Geometry: final body of the model. Coordinates: model frame, mm. Face numbers are marked on the shaded views. A direction names the side the tool comes from. Give positions to 0.01 mm unless a question says otherwise; leave off trailing zeros. Loops run counter-clockwise (first coordinate to the right, second up) from the corner with the lowest first, then second, coordinate; pieces in that order, holes last.
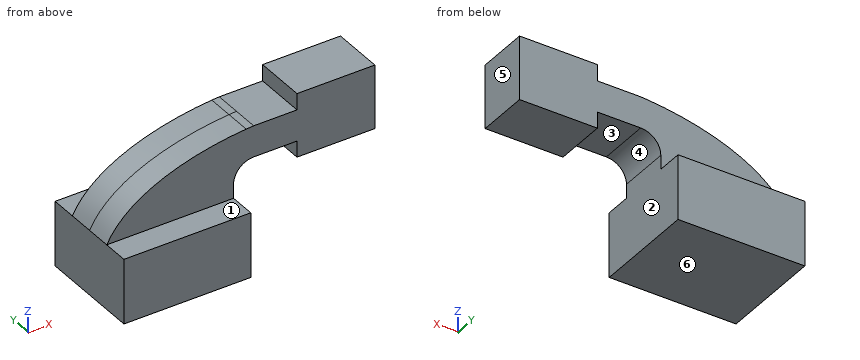
```python
from build123d import *

# Parameters (mm, degrees)
F1_DEPTH = 12.5
F2_DEPTH = 25
F0_W     = 18.6651162803
F0_H     = 7.8595249355
F0_H_2   = 15
F0_H_3   = 7.7596530318
F3_DEPTH = 12.5


with BuildPart() as f1:
    # F0 (on Front) → F1 (new body, symmetric)
    with BuildSketch(Plane.XZ):
        with BuildLine():
            add(Edge.make_bspline(
                [(-60.8189068735, 31.1434771866), (-50.2214631846, 51.7385184087), (-18.8444322176, 60.1326987931), (6.0483806323, 62.2375197437)],
                knots=[0, 0, 0, 0, 73.5359127192, 73.5359127192, 73.5359127192, 73.5359127192], degree=3))
            Line((-60.8189068735, 31.1434771866), (-15, 31.1434771866))
            Line((-15, 31.1434771866), (-15, 37.8545261919))
            ThreePointArc((-15, 37.8545261919), (-9.0100386658, 53.9601517758), (6.0483806323, 62.2375197437))
        make_face()
        with BuildLine():
            Line((-15, 31.1434771866), (0, 31.1434771866))
            Line((0, 31.1434771866), (0, 37.8545261919))
            ThreePointArc((0, 37.8545261919), (2.8255814232, 44.6760831855), (9.6471384168, 47.5016646087))
            Line((9.6471384168, 47.5016646087), (30.4094552994, 47.5016646087))
            Line((30.4094552994, 47.5016646087), (30.4094552994, 62.5016646087))
            Line((30.4094552994, 62.5016646087), (9.6471384168, 62.5016646087))
            add(Edge.make_bspline(
                [(6.0483806323, 62.2375197437), (7.2645024211, 62.3403493691), (8.4651480287, 62.4281678914), (9.6471384168, 62.5016646087)],
                knots=[73.5359127192, 73.5359127192, 73.5359127192, 73.5359127192, 77.1284607473, 77.1284607473, 77.1284607473, 77.1284607473], degree=3))
            ThreePointArc((6.0483806323, 62.2375197437), (-9.0100386658, 53.9601517758), (-15, 37.8545261919))
            Line((-15, 37.8545261919), (-15, 31.1434771866))
        make_face()
    extrude(amount=F1_DEPTH, both=True)

    # F0 (on Front) → F2 (join, symmetric)
    with BuildSketch(Plane.XZ):
        Polygon((-60.8189068735, 0), (0, 0), (0, 31.1434771866), (-15, 31.1434771866), (-60.8189068735, 31.1434771866), align=None)
    extrude(amount=F2_DEPTH, both=True)

    # F0 (on Front) → F3 (join, symmetric)
    with BuildSketch(Plane.XZ):
        with Locations((39.7420134395, 66.4314270765)):
            Rectangle(F0_W, F0_H)
        with Locations((39.7420134395, 55.0016646087)):
            Rectangle(F0_W, F0_H_2)
        with Locations((39.7420134395, 43.6218380928)):
            Rectangle(F0_W, F0_H_3)
        Polygon((49.0745715797, 62.5016646087), (49.0745715797, 47.5016646087), (49.0745715797, 39.7420115769), (67.73968786, 39.7420115769), (67.73968786, 70.3611895442), (49.0745715797, 70.3611895442), align=None)
    extrude(amount=F3_DEPTH, both=True)


solid = f1.part
```
Q1. Mould query, pull axis X, two halves, no side actions, for the marked faces 4, 5 and 6. Classes: +X half, -X half, draft (parallel to the pull), parting line (faces both ways), or undercut.
Q2. Section query A-A, the plane x = 27.5. Return loops of the section in (y, z).
Q3. Section query B-B, the plane z = 7. Return loops of the section in (x, y), and give its area (3 significant figures).
Q4. Reachability of the marked faces 1, 2 and 3 from +Z, -Z, +X, -X, +Y, -Y: full face, straight path, thin tool, end or side. Return the list, or none.
Q5. Pin query (flat end, axial travel): pin 1 Ø11.5 at (y, z) = (9, 18) entering from +X; pin 2 Ø4 at (y, z) = (-5, 43.5) entering from -X; pin 3 Ø4 at (x, y) = (-21, -20) entering from +Z. Return the tip coordinate at first contact, or that it passes through.
Q6. Material intervals for probe 1 along Y at (x, z) = (48.5, 55); probe 2 along X at (y, z) = (-21, 24.5); probe 3 along Z at (x, y) = (28, -7), sorted ascending.
Resolved:
1. face 4: undercut
1. face 5: +X half
1. face 6: draft
2. outline: (-12.5, 47.5) - (12.5, 47.5) - (12.5, 62.5) - (-12.5, 62.5) - close
3. outline: (-60.82, -25) - (0, -25) - (0, 25) - (-60.82, 25) - close
3. area: 3,040 mm2
4. face 1: +Z, +X, -X, -Y
4. face 2: -Z, +X, +Y, -Y
4. face 3: -Z, +Y, -Y
5. pin 1: stops at x = 0
5. pin 2: stops at x = -52.82
5. pin 3: stops at z = 31.14
6. probe 1: y = -12.5 to 12.5
6. probe 2: x = -60.82 to 0
6. probe 3: z = 47.5 to 62.5
